Autodesk Inventor part; units mm, degrees
ref_plane "YZ Plane" through (0, 0, 0) normal (1, 0, 0) x (0, 1, 0)
ref_plane "XZ Plane" through (0, 0, 0) normal (0, 1, 0) x (-1, 0, 0)
ref_plane "XY Plane" through (0, 0, 0) normal (0, 0, 1) x (1, 0, 0)
sketch "Skizze3" plane through (0, 0, 0) normal (0, 0, 1) x (1, 0, 0)
  line L0 (0, 0) -> (-120, 0) construction
  line L1 (0, 10) -> (-120, 10)
  line L2 (-120, -10) -> (0, -10)
  arc A0 (0, -10) -> (0, 10) centre (0, 0) ccw
  arc A1 (-120, 10) -> (-120, -10) centre (-120, 0) ccw
  circle A2 centre (0, 0) radius 5
  circle A3 centre (-120, 0) radius 2.75
  circle A4 centre (0, 0) radius 4.5
  point P0 (-60, 0)
  dimension "d4" = 120
  dimension "d5" = 20
  dimension "d6" = 10
  dimension "d7" = 5.5
  dimension "d12" = 9
extrude "Extrusion3" add sketch "Skizze3" along normal blind 5 contours A0 L2 A1 L1
extrude "Extrusion4" add sketch "Skizze3" along normal blind 1 contours A2
equation "\"d4\" = Gelenk_einfach"
equation "\"Gelenk_einfach\" = 120"
properties part number "BT001_trajan20_21" material "Kunststoff, undurchsichtig Schwarz"
Verification items for the finished model (mm, model axes). A direction names the side the tool comes from. Give positions to 0.01 mm unless a question says otherwise; leave off trailing zeros. Write each loop counter-clockwise with the first axis right and the second up, starting at its lowest first coordinate (ties: lowest second). Pieces come first, ordered by that corner, then holes. Notation, with made-up numbers: M 83,83 L 114,83 A13 cw 114,90 Z; hole C -28.5,9.25 d2. An arc over 180 degrees is marked long. Use CSV: the item, a comma, the result in double quotes.
1) Go/stop test with a flat-tipped pin: pin 1 Ø6.5 at (x, y) = (-120, 0) entering from -Z. Record where the tip stops, or that it passes through.
Final values:
pin 1,"z = 0"
2) Cross-section at C-C (y = 6.5). Enter the section's corners in (x, z).
Final values:
outline,"M -127.6,0 L 7.6,0 L 7.6,5 L -127.6,5 Z"
3) Release check for a two-part mould opening along X. For faces 3 (the face through (-0.59, -4.46, 0.49)), 4 (the face through (-120.596, 2.685, 2.465)), 5 (the face through (10, 0, 2)), 6 (the face through (-130, 0, 2)) record: released by +X, released by -X, zero draft, split by the parting line, or undercut.
Final values:
face 3,"undercut"
face 4,"undercut"
face 5,"released by +X"
face 6,"released by -X"
4) Cross-section at A-A (y = 0). Enter the section's corners in (x, z).
Final values:
outline,"M -130,0 L -122.75,0 L -122.75,5 L -130,5 Z; M -117.25,0 L -4.5,0 L -4.5,1 L -5,1 L -5,5 L -117.25,5 Z; M 4.5,0 L 10,0 L 10,5 L 5,5 L 5,1 L 4.5,1 Z"
5) Material ranges on line 1 along X through (y, z) = (0.25, 2.1); line 2 along X through (y, z) = (-2.5, 3.6); line 3 along Y through (x, z) = (0, 0.75), recorded low to high.
Final values:
line 1,"-130 to -122.74, -117.26 to -4.99, 4.99 to 10"
line 2,"-129.68 to -121.15, -118.85 to -4.33, 4.33 to 9.68"
line 3,"-10 to -4.5, 4.5 to 10"
6) Access from +Z, -Z, +X, -X, +Y, -Y to the whole of each face (thin tool, end or side, straight path). Record for faces 1 (the face through (-61, 0, 5)), 2 (the face through (-1.08, 4.88, 2.97)).
Final values:
face 1,"+Z, +X, -X, +Y, -Y"
face 2,"+Z"
7) Cross-section at B-B (z = 3.25). Enter the section's corners in (x, y), plus the area to 3 significant figures.
Final values:
outline,"M -120,-10 L 0,-10 A10 ccw 0,10 L -120,10 A10 ccw Z; hole C -120,0 d5.5; hole C 0,0 d10"
area,"2,610 mm²"
